Build history of the part. All positions in model axes, mm. Face numbers are marked on the shaded views. A direction names the side the tool comes from. Coordinates: 2 decimals unless noted, no trailing zeros. Loops run counter-clockwise (first coordinate to the right, second up) from the corner with the lowest first, then second, coordinate; pieces in that order, holes last.
Item 1: Cut at B-B (z = 1). List the corners of the cut face in (x, y), and give its area (3 significant figures).
Item 2: Cut at A-A (y = 1). List the corners of the cut face in (x, z), and give its area (3 significant figures).
Item 3: Drill centre lines: line 1 along X through (y, z) = (0.6, 0); line 2 along Z through (x, y) = (14.5, 0.95); line 3 along X through (y, z) = (2.1, 13). Where is each one in solid material? Low to high.
Item 4: Cut at D-D (z = 5.75). List the corners of the cut face in (x, y), and give its area (3 significant figures).
Item 5: Mould opens along Z. For the marked faces 1, 2, 3 and 4 say: released by +Z, released by -Z, zero draft, split by the parting line, or undercut.
Item 6: 3-axis set-ups, long thin cutter, end or side, ignore diameter. For the marked faces 5 and 6: which of +Z, -Z, +X, -X, +Y, -Y reach the whole face in a straight line?
Item 7: Cut at C-C (x = 14.5). List the corners of the cut face in (y, z).
Item 8: Flat gauge pins, fed straight in: pin 1 (1.5 mm diameter, centred on x = 10, z = 7, fed in from +Y); pin 2 (1.5 mm diameter, centred on x = 8, y = 1.5, fed in from +Z); pin 3 (1 mm diameter, centred on y = 1.5, z = 1.5, fed in from +X). Where does each tip first touch, or does it go through?
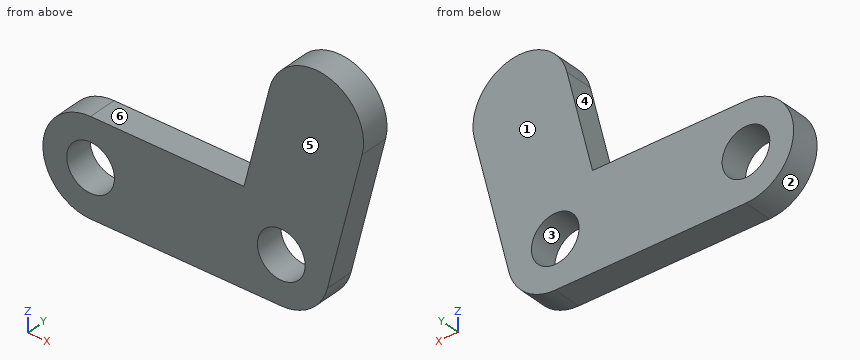
from build123d import *

# Parameters (mm, degrees)
SKETCH1_R           = 2.5
BOSS_EXTRUDE1_DEPTH = 3


with BuildPart() as part:
    # Sketch1 → Boss-Extrude1 (new body)
    # profile 1 of 3: a face of its own
    with BuildSketch(Plane(origin=(0, 0, 0), x_dir=(1, 0, 0), z_dir=(0, 1, 0))):
        with BuildLine():
            Line((20, 5), (0, 5))
            ThreePointArc((0, 5), (-5, 0), (0, -5))
            Line((0, -5), (16.093571867, -5))
            Line((16.093571867, -5), (15.148521369, -1.209609478))
            ThreePointArc((15.148521369, -1.209609478), (16.059946232, 3.078307377), (20, 5))
        make_face()
        with Locations(Location((0, 0, 0), (0, 0, 270))):
            Circle(SKETCH1_R, mode=Mode.SUBTRACT)
    # profile 2 of 3: a face of its own
    with BuildSketch(Plane(origin=(0, 0, 0), x_dir=(1, 0, 0), z_dir=(0, 1, 0))):
        with BuildLine():
            ThreePointArc((24.851478631, 1.209609478), (23.078307377, 3.940053768), (20, 5))
            ThreePointArc((20, 5), (16.059946232, 3.078307377), (15.148521369, -1.209609478))
            Line((15.148521369, -1.209609478), (16.093571867, -5))
            Line((16.093571867, -5), (20, -5))
            ThreePointArc((20, -5), (23.940053768, -3.078307377), (24.851478631, 1.209609478))
        make_face()
        with Locations(Location((20, 0, 0), (0, 0, 270))):
            Circle(SKETCH1_R, mode=Mode.SUBTRACT)
    # profile 3 of 3: a face of its own
    with BuildSketch(Plane(origin=(0, 0, 0), x_dir=(1, 0, 0), z_dir=(0, 1, 0))):
        with BuildLine():
            Line((28.480307065, -13.344826416), (24.851478631, 1.209609478))
            ThreePointArc((24.851478631, 1.209609478), (23.940053768, -3.078307377), (20, -5))
            Line((20, -5), (16.093571867, -5))
            Line((16.093571867, -5), (18.777349803, -15.764045372))
            ThreePointArc((18.777349803, -15.764045372), (24.838437912, -19.405914526), (28.480307065, -13.344826416))
        make_face()
    extrude(amount=BOSS_EXTRUDE1_DEPTH)


solid = part.part
Filled sheet:
1. outline: (-4.9, 0) - (-2.29, 0) - (-2.29, 3) - (-4.9, 3) - close; (2.29, 0) - (17.71, 0) - (17.71, 3) - (2.29, 3) - close; (22.29, 0) - (25.4, 0) - (25.4, 3) - (22.29, 3) - close
1. area: 63.4 mm2
2. outline: (0, -5) - (20, -5) arc R5 ccw to (24.85, -1.21) - (28.48, 13.34) arc R5 ccw to (18.78, 15.76) - (16.09, 5) - (0, 5) arc R5 ccw to start; hole circle Ø5 at (0, 0); hole circle Ø5 at (20, 0)
2. area: 386 mm2
3. line 1: x = -5 to -2.5, 2.5 to 17.5, 22.5 to 25.15
3. line 2: z = -5 to 5
3. line 3: x = 18.09 to 28.39
4. outline: (16.28, 0) - (26.59, 0) - (26.59, 3) - (16.28, 3) - close
4. area: 30.9 mm2
5. face 1: zero draft
5. face 2: split by the parting line
5. face 3: undercut
5. face 4: released by +Z
6. face 5: +Z, -Z, +X, -X, -Y
6. face 6: +Z, -X, +Y, -Y
7. outline: (0, -5) - (3, -5) - (3, 5) - (0, 5) - close
8. pin 1: passes through
8. pin 2: stops at z = 5
8. pin 3: stops at x = 25.65
